Could you check a few things on this model? Use its own coordinates, in mm. A direction names the side the tool comes from. Give positions to 0.01 mm unless a question says otherwise; leave off trailing zeros. Loops run counter-clockwise (first coordinate to the right, second up) from the corner with the lowest first, then second, coordinate; pieces in that order, holes last.
1. Imagine slicing it at B-B (x = 0). List the corners of the cut face in (y, z) for me, plus the area to 3 significant figures.
2. Imagine slicing it at D-D (y = 0). List the corners of the cut face in (x, z) for me, plus the area to 3 significant figures.
3. I need wall thicknesses on line 1 along Y through (x, z) = (0, 2.5); line 2 along Y through (x, z) = (0, 3.25); line 3 along Z through (x, y) = (-3.5, -2.25). Which ranges of each line are inside material? Lowest first, please.
4. Imagine slicing it at A-A (z = 0). List the corners of the cut face in (x, y) for me, plus the area to 3 significant figures.
5. For P1, Ø5, axis at x = 2.5, z = -3.5, coming from the -Y side; P2, Ø1.5, axis at y = -2.5, z = 1.5, coming from the +X side; P3, Ø1, axis at y = -5.5, z = 2, coming from the +X side, each with a flat end and sliding along its axis, tell me the tip position at first contact or that it passes through.
6. For faces 1 (the flat face through (0, -8.35, 0)), 2 (the cylindrical face through (0, -6, -2)), which set-ups out of +Z, -Z, +X, -X, +Y, -Y let a thin tool reach every point of the face, with its end or its side?
7. Imagine slicing it at C-C (y = -6.75). List the corners of the cut face in (x, z) for me.
```python
from build123d import *

# Parameters (mm, degrees)
SKIZZE2_R                       = 2
AUFSATZ_LINEAR_AUSTRAGEN1_DEPTH = 5
FASE1_SIZE                      = 0.6


with BuildPart() as part:
    # Skizze1 → Rotation1 (revolve)
    with BuildSketch(Plane(origin=(0, 0, 0), x_dir=(0, 0, -1), z_dir=(1, 0, 0))):
        with BuildLine():
            Line((0, 4.85), (0, -3.35))
            Line((0, -3.35), (3.507135583, -3.35))
            ThreePointArc((3.507135583, -3.35), (4.459260028, 1.907223112), (0, 4.85))
        make_face()
    revolve(axis=Axis((0, 21.112600536, 0), (0, -1, 0)))

    # Skizze2 → Aufsatz-Linear austragen1 (add)
    with BuildSketch(Plane.XZ.offset(3.35)):
        Circle(SKIZZE2_R)
    extrude(amount=AUFSATZ_LINEAR_AUSTRAGEN1_DEPTH)

    # Fase1
    fase1_edges = [part.edges().sort_by_distance(p)[0] for p in [
        (-2, -8.35, 0),
    ]]
    chamfer(fase1_edges, length=FASE1_SIZE)


solid = part.part
```
Derived:
1. outline: (-8.35, -1.4) - (-7.75, -2) - (-3.35, -2) - (-3.35, -3.51) arc R4.85 ccw (long way) to (-3.35, 3.51) - (-3.35, 2) - (-7.75, 2) - (-8.35, 1.4) - close
1. area: 86.3 mm2
2. outline: circle Ø9.7 at (0, 0)
2. area: 73.9 mm2
3. line 1: y = -3.35 to 4.16
3. line 2: y = -3.35 to 3.6
3. line 3: z = -2.49 to 2.49
4. outline: (-3.51, -3.35) - (-2, -3.35) - (-2, -7.75) - (-1.4, -8.35) - (1.4, -8.35) - (2, -7.75) - (2, -3.35) - (3.51, -3.35) arc R4.85 ccw (long way) to start
4. area: 86.3 mm2
5. P1: stops at y = -7.95
5. P2: stops at x = 4.34
5. P3: stops at x = 1.32
6. face 1: +Z, -Z, +X, -X, -Y
6. face 2: -Y
7. outline: circle Ø4 at (0, 0)
